Model file for the job. Use its own axes, mm. A direction names the side the tool comes from. Give positions to 0.01 mm unless a question says otherwise; leave off trailing zeros. Write each loop counter-clockwise with the first axis right and the second up, starting at its lowest first coordinate (ties: lowest second). Pieces come first, ordered by that corner, then holes. Notation, with made-up numbers: M 57.25,31.25 L 107.25,31.25 A21 cw 107.25,44.25 Z; hole C 42.5,-11 d9. An arc over 180 degrees is marked long. Answer as a JSON object with one key per item and string values. Group by question number.
```python
from build123d import *

# Parameters (mm, degrees)
CYLINDER001_R     = 2
CYLINDER001_DEPTH = 10
CYLINDER_R        = 2
CYLINDER_DEPTH    = 10
EXTRUDE_DEPTH     = 12


with BuildPart() as cylinder001:
    # Cylinder001 → Cylinder001 (new body)
    with BuildSketch(Plane(origin=(39, 13, 6), x_dir=(1, 0, 0), z_dir=(0, -1, 0))):
        Circle(CYLINDER001_R)
    extrude(amount=CYLINDER001_DEPTH)


with BuildPart() as cylinder:
    # Cylinder → Cylinder (new body)
    with BuildSketch(Plane(origin=(-39, 13, 6), x_dir=(1, 0, 0), z_dir=(0, -1, 0))):
        Circle(CYLINDER_R)
    extrude(amount=CYLINDER_DEPTH)


with BuildPart() as cut001:
    # Sketch → Extrude (new body)
    with BuildSketch(Plane.XY):
        Polygon((-29, -16.5), (29, -16.5), (29, 10), (45, 10), (45, 6), (33, 6), (33, -20.5), (-33, -20.5), (-33, 6), (-45, 6), (-45, 10), (-29, 10), align=None)
    extrude(amount=EXTRUDE_DEPTH)

    # Cut: cut Cylinder
    add(cylinder.part, mode=Mode.SUBTRACT)

    # Cut001: cut Cylinder001
    add(cylinder001.part, mode=Mode.SUBTRACT)


solid = cut001.part
```
Q1. Wall check: L1, parallel to X at y = 7.7, z = 6; L2, parallel to X at y = -8, z = 2.75; L3, parallel to Z at x = -39, y = 7.85. Give the ranges that are in metal, low to high.
Q2. Slice it at C-C, the plane z = 1.5. Write the cut outline in (x, y).
Q3. Slice it at B-B, the plane x = -39. Write the cut outline in (y, z), then the cut area to 3 significant figures.
Q4. Slice it at A-A, the plane z = 6. Write the cut outline in (x, y), then the cut area to 3 significant figures.
Q5. Slice it at D-D, the plane x = -8. Write the cut outline in (y, z).
Q6. 3-axis set-ups, long thin cutter, end or side, ignore diameter. For faces 1 (the flat face through (-33, -7, 6)), 2 (the flat face through (39, 6, 3)), 3 (the flat face through (0, -16.5, 6)): which of +Z, -Z, +X, -X, +Y, -Y reach the whole face in a straight line?
Q7. Drop flat-ended pins along their axis: P1, Ø6, axis at y = -9, z = 6.5, coming from the -X side; P2, Ø3.5, axis at x = 41, z = 5, coming from the -Y side; P3, Ø3, axis at x = 39, z = 6, coming from the -Y side. Give the stop position or say it passes through.
Q8. Two-plate mould, pull along Z, no slides. Class faces 4 (the flat face through (0, -19, 12)), 5 (the cylindrical face through (-41, 8, 6)), 6 (the flat face through (29, -3, 6)), 7 (the flat face through (0, -19, 0)): +Z half, -Z half, draft (parallel to the pull), parting line (faces both ways), or undercut.
Solved:
{
 "1": {"L1": "x = -45 to -41, -37 to -29, 29 to 37, 41 to 45", "L2": "x = -33 to -29, 29 to 33", "L3": "z = 0 to 4, 8 to 12"},
 "2": {"outline": "M -45,6 L -33,6 L -33,-20.5 L 33,-20.5 L 33,6 L 45,6 L 45,10 L 29,10 L 29,-16.5 L -29,-16.5 L -29,10 L -45,10 Z"},
 "3": {"outline": "M 6,0 L 10,0 L 10,4 L 6,4 Z; M 6,8 L 10,8 L 10,12 L 6,12 Z", "area": "32.0 mm²"},
 "4": {"outline": "M -45,6 L -41,6 L -41,10 L -45,10 Z; M -37,6 L -33,6 L -33,-20.5 L 33,-20.5 L 33,6 L 37,6 L 37,10 L 29,10 L 29,-16.5 L -29,-16.5 L -29,10 L -37,10 Z; M 41,6 L 45,6 L 45,10 L 41,10 Z", "area": "540 mm²"},
 "5": {"outline": "M -20.5,0 L -16.5,0 L -16.5,12 L -20.5,12 Z"},
 "6": {"face 1": "+Z, -Z, -X, -Y", "face 2": "+Z, -Z, +X, -Y", "face 3": "+Z, -Z, +Y"},
 "7": {"P1": "stops at x = -33", "P2": "stops at y = 6", "P3": "passes through"},
 "8": {"face 4": "+Z half", "face 5": "undercut", "face 6": "draft", "face 7": "-Z half"}
}
